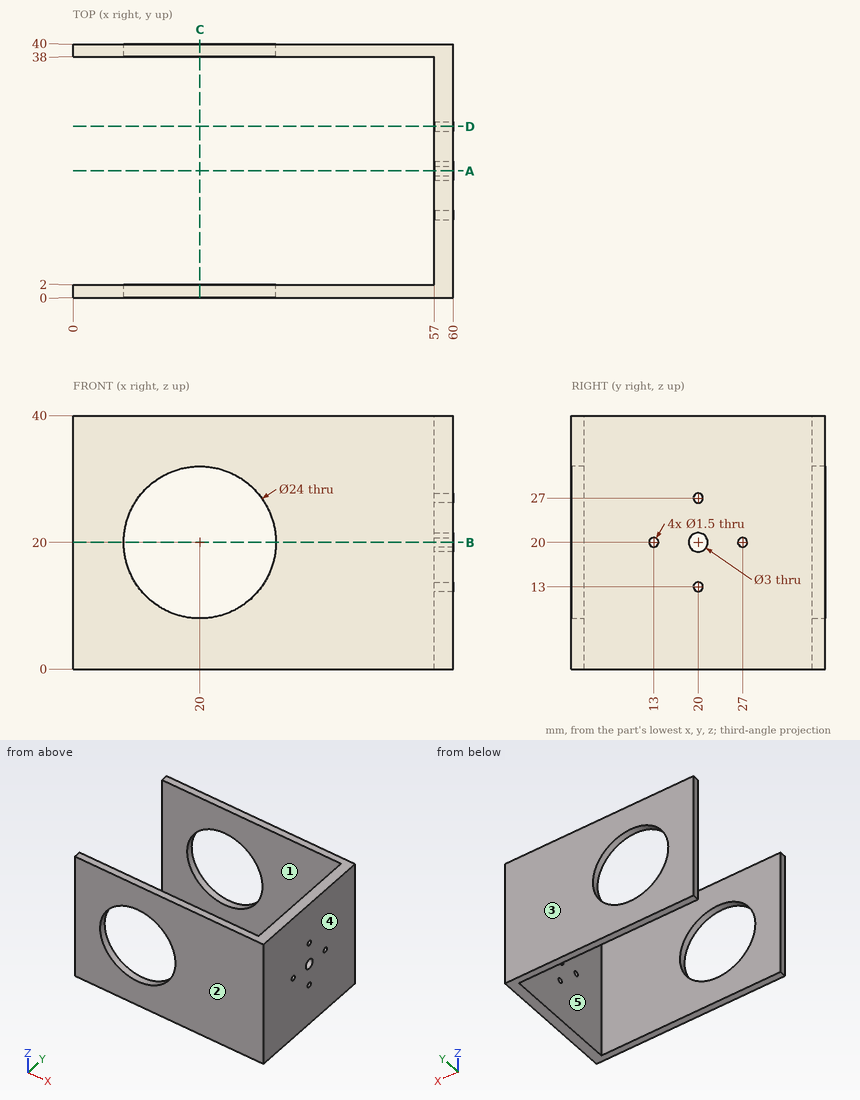
The figure shows three views and two pictorial views of one solid part (mm, origin at its lowest corner). Answer the questions. A direction names the side the tool comes from. Give positions to 0.01 mm unless a question says otherwise; leave off trailing zeros. Loops run counter-clockwise (first coordinate to the right, second up) from the corner with the lowest first, then second, coordinate; pieces in that order, holes last. Notation, with made-up numbers: (41, 54.25) - (56, 54.25) arc R14 cw to (56, 73.25) - close; hole circle Ø11 at (-20.5, 64). An arc over 180 degrees is marked (long way). Use one line per item in the form item = value.
1. The mould has two halves that part along Y. Classify the marked faces 3, 4 and 5: pulls with the +Y half, pulls with the -Y half, needs draft (parallel to the pull), parting line crosses it, or undercut.
Calculated:
face_3 = pulls with the +Y half
face_4 = needs draft
face_5 = undercut
2. Section A-A on y = 20 is taken. Give the vertices of the cut face in (x, z), then the cut area to 3 significant figures.
Calculated:
outline = (57, 0) - (60, 0) - (60, 12.25) - (57, 12.25) - close; (57, 13.75) - (60, 13.75) - (60, 18.5) - (57, 18.5) - close; (57, 21.5) - (60, 21.5) - (60, 26.25) - (57, 26.25) - close; (57, 27.75) - (60, 27.75) - (60, 40) - (57, 40) - close
area = 102 mm^2
3. Which of the six approach directions +Z, -Z, +X, -X, +Y, -Y give full straight-line access (tool end or side, diameter ignored) to the marked faces 1 and 2?
Calculated:
face_1 = +Z, -Z, -X
face_2 = +Z, -Z, +X, -X, -Y
4. Find the intervals of material crossed by line 1 along Y through (x, z) = (57.6, 20); line 2 along Y through (x, z) = (44, 8); line 3 along X through (y, z) = (33.5, 33), in increasing order. Write a range as [from, to].
Calculated:
line_1 = [0, 12.25], [13.75, 18.5], [21.5, 26.25], [27.75, 40]
line_2 = [0, 2], [38, 40]
line_3 = [57, 60]
5. Section B-B on z = 20 is taken. Give the vertices of the cut face in (x, y).
Calculated:
outline = (0, 0) - (8, 0) - (8, 2) - (0, 2) - close; (0, 38) - (8, 38) - (8, 40) - (0, 40) - close; (32, 0) - (60, 0) - (60, 12.25) - (57, 12.25) - (57, 2) - (32, 2) - close; (32, 38) - (57, 38) - (57, 27.75) - (60, 27.75) - (60, 40) - (32, 40) - close; (57, 13.75) - (60, 13.75) - (60, 18.5) - (57, 18.5) - close; (57, 21.5) - (60, 21.5) - (60, 26.25) - (57, 26.25) - close
6. Section D-D on y = 27 is taken. Give the vertices of the cut face in (x, z), then the cut area to 4 significant figures.
Calculated:
outline = (57, 0) - (60, 0) - (60, 19.25) - (57, 19.25) - close; (57, 20.75) - (60, 20.75) - (60, 40) - (57, 40) - close
area = 115.5 mm^2
7. Section C-C on x = 20 is taken. Give the vertices of the cut face in (y, z), then the cut area to 3 significant figures.
Calculated:
outline = (0, 0) - (2, 0) - (2, 8) - (0, 8) - close; (0, 32) - (2, 32) - (2, 40) - (0, 40) - close; (38, 0) - (40, 0) - (40, 8) - (38, 8) - close; (38, 32) - (40, 32) - (40, 40) - (38, 40) - close
area = 64.0 mm^2
8. Given pin 1 Ø12 at (x, z) = (24.5, 18.5) entering from +Y; pin 2 Ø6 at (y, z) = (12.5, 28) entering from -X, each flat-ended and moving along its own axis, determine where each tip first touches the part or whether it passes through.
Calculated:
pin_1 = through
pin_2 = 57
